The listing builds one solid part. Answer for the finished solid, in the listing's coordinates (mm). Face numbers are marked on the shaded views. A direction names the side the tool comes from. Give positions to 0.01 mm unless a question says otherwise; leave off trailing zeros. Loops run counter-clockwise (first coordinate to the right, second up) from the corner with the lowest first, then second, coordinate; pieces in that order, holes last.
Item 1: Section C-C, the plane y = 43 is taken. Give the vertices of the cut face in (x, z).
Item 2: Section D-D, the plane z = 16 is taken. Give the vertices of the cut face in (x, y), and give its area (3 significant figures).
Item 3: Each of these flat-tipped pins is pushed along its axis until it touches: pin 1 Ø3.5 at (x, z) = (-7, 28) entering from -Y; pin 2 Ø5 at (x, z) = (-4, -2) entering from +Y; pin 3 Ø11 at (x, z) = (-6, 24.5) entering from +Y; pin 4 Ø3 at (x, z) = (0.5, 9.5) entering from +Y. Where does it stop, or does it pass through?
Item 4: Consider line 1 along Z through (x, y) = (7.5, 33); line 2 along X through (y, z) = (40, 27); line 3 along Z through (x, y) = (0, 0.95). Determine where each line is inside the solid, lowest interval first.
Item 5: The mould has two halves that part along Y. Classify the marked faces 1, 2, 3 and 4: pulls with the +Y half, pulls with the -Y half, needs draft (parallel to the pull), parting line crosses it, or undercut.
Item 6: Section A-A, the plane y = 8 is taken. Give the vertices of the cut face in (x, z), and give its area (3 significant figures).
Item 7: A tool of negligible diameter and unlimited length cuts with its end or side. For the marked faces 5, 6, 7 and 8, from which of +Z, -Z, +X, -X, +Y, -Y can it reach the whole face along a straight path? Write none if from no direction.
Item 8: Section B-B, the plane x = -3.5 is taken. Give the vertices of the cut face in (y, z).
Autodesk Inventor part; units mm, degrees
ref_plane "YZ Plane" through (0, 0, 0) normal (1, 0, 0) x (0, 1, 0)
ref_plane "XZ Plane" through (0, 0, 0) normal (0, 1, 0) x (-1, 0, 0)
ref_plane "XY Plane" through (0, 0, 0) normal (0, 0, 1) x (1, 0, 0)
sketch "Sketch1" plane through (0, 0, 0) normal (0, 1, 0) x (-1, 0, 0)
  line L0 (10, 31.05) -> (-10, 31.05)
  line L1 (-10, 31.05) -> (-10, -10)
  line L2 (-10, -10) -> (10, -10)
  line L3 (10, -10) -> (10, 31.05)
  point P0 (0, 0)
  dimension "d0" = 20
  dimension "d1" = 41.05
extrude "Extrusion1" add sketch "Sketch1" along normal blind 2
sketch "Sketch2" plane through (0, 2, 0) normal (0, 1, 0) x (1, 0, 0)
  line L0 (-10, -31.05) -> (10, -31.05)
  line L1 (0, -31.05) -> (-6.35, -31.05)
  line L2 (-6.35, -20.15) -> (6.35, -20.15)
  line L3 (6.35, -31.05) -> (0, -31.05)
  line L4 (10, 10) -> (-10, 10)
  line L5 (-6.35, -0.9) -> (6.35, -0.9)
  line L6 (-6.35, 10) -> (6.35, 10)
  line L7 (-6.35, -31.05) -> (-10, -31.05)
  line L8 (-10, 10) -> (-10, -31.05)
  line L9 (-10, -20.15) -> (-6.35, -20.15)
  line L10 (6.35, -31.05) -> (10, -31.05)
  line L11 (10, -31.05) -> (10, 10)
  line L12 (10, -20.15) -> (6.35, -20.15)
  line L13 (6.35, -0.9) -> (10, -0.9)
  line L14 (10, 10) -> (6.35, 10)
  line L15 (10, -0.9) -> (10, 10)
  line L16 (10, -31.05) -> (10, -20.15)
  line L17 (-10, -31.05) -> (-10, -20.15)
  line L18 (-6.35, -0.9) -> (-10, -0.9)
  line L19 (-10, -0.9) -> (-10, 10)
  line L20 (-10, 10) -> (-6.35, 10)
  point P0 (0, 0)
  dimension "d4" = 6.35
  dimension "d5" = 10.9
  dimension "d6" = 12.7
  dimension "d7" = 10.9
extrude "Extrusion2" add sketch "Sketch2" along normal blind 48.3354 contours L8 L9 L2 L12 L11 L0 | L8 L4 L11 L13 L5 L18
sketch "Sketch9" plane through (-10, 0, 31.05) normal (0, 0, 1) x (1, 0, 0)
  arc A0 (15.084, 42.3223) -> (4.684, 42.3223) centre (9.884, 42.3223) ccw
  line L0 (15.084, 35.9247) -> (15.084, 42.3223)
  line L1 (4.684, 41.1247) -> (4.684, 42.3223)
  arc A1 (15.084, 42.3223) -> (4.684, 42.3223) centre (9.884, 42.3223) ccw
  line L2 (4.684, 42.3223) -> (4.684, 35.9247)
  line L3 (9.8827, 20.3222) -> (-0.0013, 20.3222)
  line L4 (-0.0013, 30.726) -> (-0.0013, 20.3222)
  line L5 (4.684, 35.9247) -> (4.684, 30.726)
  line L6 (15.084, 35.9247) -> (15.0853, 25.5254)
  arc A2 (15.084, 35.9247) -> (15.084, 35.9251) centre (9.884, 35.9243) ccw
  line L7 (4.684, 30.726) -> (-0.0013, 30.726)
  arc A3 (9.8827, 20.3222) -> (15.0853, 25.5254) centre (9.8827, 25.5248) ccw
  point P0 (10, 0)
fillet "Fillet4" radius 10 4 edges at (10, 50.3354, 25.6) (-10, 50.3354, 25.6) (-10, 50.3354, -4.55) (10, 50.3354, -4.55)
sketch "Sketch10" plane through (0, 2, 0) normal (0, 1, 0) x (1, 0, 0)
  line L0 (10, -31.05) -> (-10, -31.05)
  line L1 (-10, 10) -> (10, 10)
  line L2 (10, -20.15) -> (10, -0.9)
  line L3 (-10, -0.9) -> (-10, -20.15)
  line L4 (10, -10.525) -> (-10, -10.525)
  circle A0 centre (0, -10.525) radius 2.125
  point P0 (0, 0)
  dimension "d53" = 41.05
  dimension "d54" = 4.25
extrude "Extrusion10" cut sketch "Sketch10" against normal blind 2
extrude "Extrusion11" cut sketch "Sketch9" against normal through all
properties part number "6 Backet Adjustment"
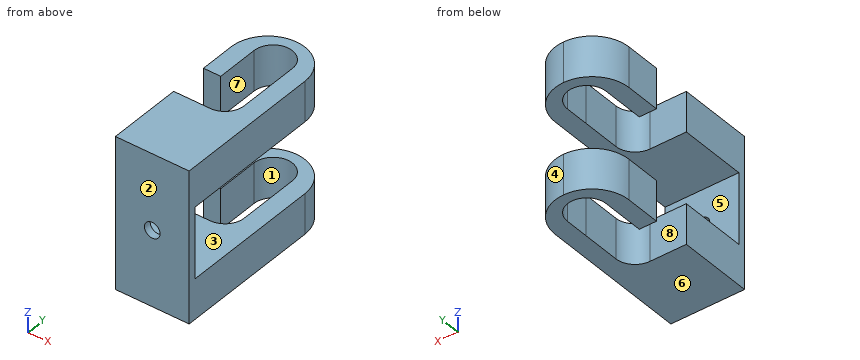
Worked answers:
1. outline: (-9.64, -10) - (-5.27, -10) - (-5.27, 0.9) - (-9.64, 0.9) - close; (-9.64, 20.15) - (-5.27, 20.15) - (-5.27, 31.05) - (-9.64, 31.05) - close; (5.04, -10) - (9.64, -10) - (9.64, 0.9) - (5.04, 0.9) - close; (5.04, 20.15) - (9.64, 20.15) - (9.64, 31.05) - (5.04, 31.05) - close
2. outline: (-10, 0) - (10, 0) - (10, 2) - (-10, 2) - close
2. area: 40.0 mm2
3. pin 1: stops at y = 0
3. pin 2: stops at y = 50.22
3. pin 3: stops at y = 50.32
3. pin 4: stops at y = 2
4. line 1: z = -10 to 0.9, 20.15 to 31.05
4. line 2: x = -10 to -5.32, 5.08 to 10
4. line 3: z = -10 to 8.4, 12.65 to 31.05
5. face 1: undercut
5. face 2: pulls with the -Y half
5. face 3: needs draft
5. face 4: pulls with the +Y half
6. outline: (-10, -10) - (10, -10) - (10, 0.9) - (-10, 0.9) - close; (-10, 20.15) - (10, 20.15) - (10, 31.05) - (-10, 31.05) - close
6. area: 436 mm2
7. face 5: +X, -X, +Y
7. face 6: -Z, +X, -X, +Y, -Y
7. face 7: +Z, -Z
7. face 8: +Z, -Z, -X
8. outline: (0, -10) - (20.32, -10) - (20.32, 0.9) - (2, 0.9) - (2, 20.15) - (20.32, 20.15) - (20.32, 31.05) - (0, 31.05) - close; (46.27, -10) - (49.7, -10) - (49.7, 0.9) - (46.27, 0.9) - close; (46.27, 20.15) - (49.7, 20.15) - (49.7, 31.05) - (46.27, 31.05) - close
